Geometry check sheet. Reference: the model listing, model coordinates, mm. A direction names the side the tool comes from. Round coordinates to 2 decimals unless told otherwise and drop trailing zeros. Use a Markdown table: item, result.
Autodesk Inventor part; units mm, degrees
ref_plane "YZ Plane" through (0, 0, 0) normal (1, 0, 0) x (0, 1, 0)
ref_plane "XZ Plane" through (0, 0, 0) normal (0, 1, 0) x (-1, 0, 0)
ref_plane "XY Plane" through (0, 0, 0) normal (0, 0, 1) x (1, 0, 0)
sketch "Sketch1" plane through (0, 0, 0) normal (0, 0, 1) x (1, 0, 0)
  circle A0 centre (0, 0) radius 75
  dimension "d0" = 150
extrude "Extrusion1" add sketch "Sketch1" along normal blind 12
sketch "Sketch2" plane through (0, 0, 12) normal (0, 0, 1) x (1, 0, 0)
  circle A0 centre (0, 0) radius 60 construction
  point P0 (60, 0)
  dimension "d3" = 120
hole "Hole1" at (60, 0, 12) direction (0, 0, -1) diameter 12 end through all
pattern_circular "Circular Pattern1" count 4 over 360 about axis through (0, 0, 0) along (0, 0, 1) of "Hole1"
sketch "Sketch3" plane through (0, 0, 12) normal (0, 0, 1) x (1, 0, 0)
  circle A0 centre (0, 0) radius 68 construction
  line L0 (48.0833, 48.0833) -> (0, 0) construction
  line L1 (0, 0) -> (75, 0) construction
  circle A1 centre (0, 0) radius 75
  dimension "d14" = 136
  dimension "d15" = 45
hole "Hole2" at (48.0833, 48.0833, 12) direction (0, 0, -1) diameter 7.2 end through all
pattern_circular "Circular Pattern2" count 4 over 360 about axis through (0, 0, 0) along (0, 0, 1) of "Hole2"
sketch "Sketch4" plane through (0, 0, 0) normal (1, 0, 0) x (0, 1, 0)
  line L0 (0, 0) -> (0, 12)
  line L1 (75, 12) -> (-75, 12)
  line L2 (75, 0) -> (-75, 0)
  line L3 (22.5, 0) -> (22.5, 8)
  line L4 (22.5, 8) -> (21, 8)
  line L5 (21, 8) -> (21, 12)
  dimension "d26" = 45
  dimension "d27" = 4
  dimension "d28" = 42
revolve "Revolution1" cut sketch "Sketch4" angle 360 about axis through (0, 0, 0) along (0, 0, 1)
chamfer "Chamfer1" distance 0.4 angle 45 4 edges at (-75, 0, 0) (-75, 0, 12) (0, -21, 12) (0, -22.5, 0)
chamfer "Chamfer2" distance 0.4 angle 45 8 edges at (-6, 60, 12) (-60, -6, 12) (6, -60, 12) (60, 6, 12) (-6, 60, 0) (-60, -6, 0) (60, 6, 0) (6, -60, 0)
properties part number "VF65-KF40-adapter" material "Stainless Steel"
(1) Thickness scan on line 1 (Y direction, x = 0, z = 3); line 2 (X direction, y = -3.5, z = 1.75); line 3 (Y direction, x = -4, z = 7.75). Record the ranges inside material, lowest first.
A:
| item | result |
|---|---|
| line 1 | y = -75 to -66, -54 to -22.5, 22.5 to 54, 66 to 75 |
| line 2 | x = -74.92 to -64.87, -55.13 to -22.23, 22.23 to 55.13, 64.87 to 74.92 |
| line 3 | y = -74.89 to -64.47, -55.53 to -22.14, 22.14 to 55.53, 64.47 to 74.89 |
(2) Release check for a two-part mould opening along X. For faces 1 (the face through (1.301, -65.857, 5.922)), 2 (the face through (-9.764, -74.362, 5.922)), 3 (the face through (16, -16, 12)), 4 (the face through (47.93, 51.68, 5.92)) record: +X half, -X half, draft (parallel to the pull), parting line (faces both ways), or undercut.
A:
| item | result |
|---|---|
| face 1 | undercut |
| face 2 | parting line |
| face 3 | draft |
| face 4 | undercut |
(3) Gauge pin test, flat ends, axial feed: pin 1 Ø10 at (x, y) = (-15.5, -11) entering from -Z; pin 2 Ø22.5 at (x, y) = (-1, 5.5) entering from -Z; pin 3 Ø5 at (y, z) = (9, 9.5) entering from -X; pin 4 Ø6 at (y, z) = (-13.5, 6) entering from -X. Record the tip position at first contact, or that the pin passes through.
A:
| item | result |
|---|---|
| pin 1 | stops at z = 0 |
| pin 2 | passes through |
| pin 3 | stops at x = -74.72 |
| pin 4 | stops at x = -74.26 |
(4) Access from +Z, -Z, +X, -X, +Y, -Y to the whole of each face (thin tool, end or side, straight path). Record for faces 5 (the face through (-6.31, 20.03, 9.83)), 6 (the face through (-7, 20, 8)).
A:
| item | result |
|---|---|
| face 5 | +Z, -Z |
| face 6 | -Z |
(5) Section check A-A on y = 0. State how many separate pieces and enclosed holes the cut face has, plus the area to 3 significant figures.
A:
| item | result |
|---|---|
| separate pieces | 4 |
| enclosed holes | 0 |
| area | 983 mm2 |
